```python
from build123d import *

# Parameters (mm, degrees)
SKETCH1_R           = 11
BOSS_EXTRUDE1_DEPTH = 4
SKETCH2_R           = 6.85
CUT_EXTRUDE1_DEPTH  = 11.96
SKETCH3_R           = 10
SKETCH3_R_2         = 8
CUT_EXTRUDE2_DEPTH  = 0.5


with BuildPart() as part:
    # Sketch1 → Boss-Extrude1 (new body, symmetric)
    with BuildSketch(Plane(origin=(0, 0, 0), x_dir=(1, 0, 0), z_dir=(0, 1, 0))):
        Circle(SKETCH1_R)
    extrude(amount=BOSS_EXTRUDE1_DEPTH, both=True)

    # Sketch2 → Cut-Extrude1 (cut)
    with BuildSketch(Plane(origin=(0, 4, 0), x_dir=(1, 0, 0), z_dir=(0, 1, 0))):
        Circle(SKETCH2_R)
    extrude(amount=-CUT_EXTRUDE1_DEPTH, mode=Mode.SUBTRACT)

    # Sketch3 → Cut-Extrude2 (cut)
    with BuildSketch(Plane(origin=(0, 4, 0), x_dir=(1, 0, 0), z_dir=(0, 1, 0))):
        Circle(SKETCH3_R)
        Circle(SKETCH3_R_2, mode=Mode.SUBTRACT)
    cut_extrude2 = extrude(amount=-CUT_EXTRUDE2_DEPTH, mode=Mode.SUBTRACT)

    # Mirror1: Cut-Extrude2 across plane
    add(cut_extrude2.mirror(Plane.ZX), mode=Mode.SUBTRACT)


solid = part.part
```
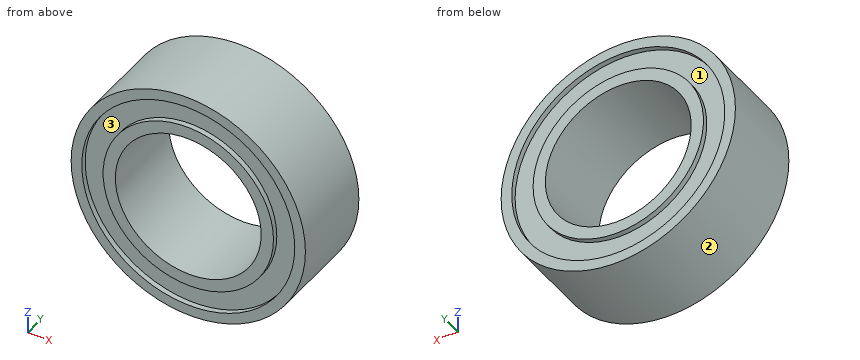
The model under review builds one solid part; all positions refer to its coordinate system, in mm. Face numbers are marked on the shaded views. Round coordinates to 2 decimals unless told otherwise and drop trailing zeros. Write each loop counter-clockwise with the first axis right and the second up, starting at its lowest first coordinate (ties: lowest second). Pieces come first, ordered by that corner, then holes. Notation, with made-up numbers: M 8.25,87.25 L 21.25,87.25 A22 ccw 21.25,111.25 Z; hole C 39.25,77.5 d7. An arc over 180 degrees is marked long. Use CSV: the item, a comma, the result in double quotes. Start each with the question number.
(1) We need section B-B, the plane x = 0. State the section outline as (y, z) points.
(2) Clearance check with flat-ended pins moving along their axes: P1, Ø6, axis at x = 2, z = -0.5, coming from the -Y side; P2, Ø2, axis at y = 2.5, z = 3, coming from the -X side; P3, Ø2, axis at x = 3, y = 2, coming from the -Z side; P4, Ø4, axis at x = -8.5, y = -2.5, coming from the -Z side. State where each tip first meets the part, or that it passes through.
(3) For line 1 along Z through (x, y) = (0, 3.7); line 2 along Z through (x, y) = (0, -0.5), list the stretches that pass through material, from the lowest coordinate up.
(4) The part is to be moulded in two halves that separate along Z. For the marked faces 1, 2 and 3, say which applies: +Z half, -Z half, draft (parallel to the pull), parting line (faces both ways), or undercut.
(5) We need section D-D, the plane z = 9.5. State the section outline as (x, y) points, then the cut area to 3 significant figures.
(6) We need section C-C, the plane y = 1. State the section outline as (x, z) points, then the cut area to 3 significant figures.
(7) We need section A-A, the plane z = 0. State the section outline as (x, y) points, then the cut area to 3 significant figures.
Findings:
1,outline,"M -4,-11 L 4,-11 L 4,-10 L 3.5,-10 L 3.5,-8 L 4,-8 L 4,-6.85 L -4,-6.85 L -4,-8 L -3.5,-8 L -3.5,-10 L -4,-10 Z; M -4,6.85 L 4,6.85 L 4,8 L 3.5,8 L 3.5,10 L 4,10 L 4,11 L -4,11 L -4,10 L -3.5,10 L -3.5,8 L -4,8 Z"
2,P1,"through"
2,P2,"x = -10.82"
2,P3,"z = -10.82"
2,P4,"z = -8.87"
3,line 1,"-11 to -10, -8 to -6.85, 6.85 to 8, 10 to 11"
3,line 2,"-11 to -6.85, 6.85 to 11"
4,face 1,"undercut"
4,face 2,"parting line"
4,face 3,"undercut"
5,outline,"M -5.55,-4 L -3.12,-4 L -3.12,-3.5 L 3.12,-3.5 L 3.12,-4 L 5.55,-4 L 5.55,4 L 3.12,4 L 3.12,3.5 L -3.12,3.5 L -3.12,4 L -5.55,4 Z"
5,area,"82.5 mm^2"
6,outline,"C 0,0 d22; hole C 0,0 d13.7"
6,area,"233 mm^2"
7,outline,"M -11,-4 L -10,-4 L -10,-3.5 L -8,-3.5 L -8,-4 L -6.85,-4 L -6.85,4 L -8,4 L -8,3.5 L -10,3.5 L -10,4 L -11,4 Z; M 6.85,-4 L 8,-4 L 8,-3.5 L 10,-3.5 L 10,-4 L 11,-4 L 11,4 L 10,4 L 10,3.5 L 8,3.5 L 8,4 L 6.85,4 Z"
7,area,"62.4 mm^2"
